Build history of the part. All positions in model axes, mm. Face numbers are marked on the shaded views. A direction names the side the tool comes from. Give positions to 0.01 mm unless a question says otherwise; leave off trailing zeros. Write each loop counter-clockwise with the first axis right and the second up, starting at its lowest first coordinate (ties: lowest second). Pieces come first, ordered by that corner, then holes.
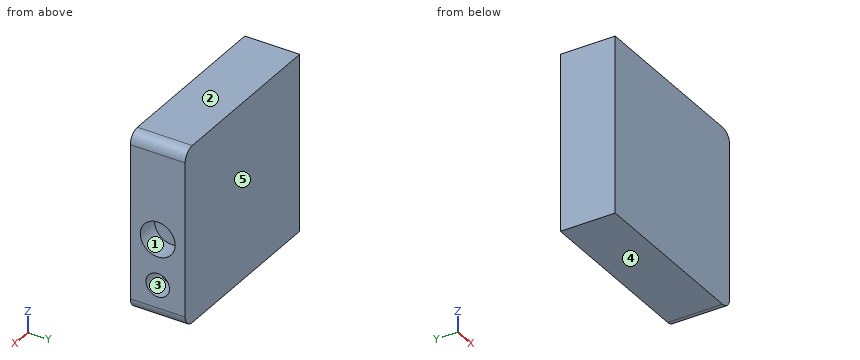
from build123d import *

# Parameters (mm, degrees)
SKETCH1_W           = 80
SKETCH1_H           = 77.5
BOSS_EXTRUDE1_DEPTH = 24
SKETCH2_R           = 5.125
SKETCH2_R_2         = 7.625
CUT_EXTRUDE1_DEPTH  = 10
FILLET1_R           = 5


with BuildPart() as part:
    # Sketch1 → Boss-Extrude1 (new body)
    with BuildSketch(Plane(origin=(0, 0, 0), x_dir=(1, 0, 0), z_dir=(0, 1, 0))):
        with Locations((40, 38.75)):
            Rectangle(SKETCH1_W, SKETCH1_H)
    extrude(amount=BOSS_EXTRUDE1_DEPTH)

    # Sketch2 → Cut-Extrude1 (cut)
    with BuildSketch(Plane(origin=(80, 0, 0), x_dir=(0, 0, -1), z_dir=(1, 0, 0))):
        with Locations((62.5, 12)):
            Circle(SKETCH2_R)
        with Locations((42.5, 12)):
            Circle(SKETCH2_R_2)
    extrude(amount=-CUT_EXTRUDE1_DEPTH, mode=Mode.SUBTRACT)

    # Fillet1
    fillet1_edges = [part.edges().sort_by_distance(p)[0] for p in [
        (80, 12, -77.5),
        (80, 12, 0),
    ]]
    fillet(fillet1_edges, radius=FILLET1_R)


solid = part.part
1. Saw through at B-B on z = -62.5. Give the cut face in (x, y) (3 decimals).
2. Drop a flat-ended pin along its axis: pin 1 (4.5 mm diameter, centred on y = 14, z = -41.5, fed in from +X). Give the stop position or say it passes through.
3. Saw through at C-C on z = -42.5. Give the cut face in (x, y) (3 decimals), plus the area to 3 significant figures.
4. Saw through at A-A on y = 12. Give the cut face in (x, z) (3 decimals).
5. Drill centre lines: line 1 along Y through (x, z) = (75, -42); line 2 along Y through (x, z) = (73, -62.5) (3 decimals); line 3 along X through (y, z) = (15.75, -39). Where is each one in solid material? Low to high.
6. 3-axis set-ups, long thin cutter, end or side, ignore diameter. For the marked faces 1 and 2: which of +Z, -Z, +X, -X, +Y, -Y reach the whole face in a straight line?
7. Mould opens along Y. For the marked faces 3, 4 and 5 say: pulls with the +Y half, pulls with the -Y half, needs draft (parallel to the pull), parting line crosses it, or undercut.
Outcome:
1. outline: (0, 0) - (80, 0) - (80, 6.875) - (70, 6.875) - (70, 17.125) - (80, 17.125) - (80, 24) - (0, 24) - close
2. pin 1: stops at x = 70
3. outline: (0, 0) - (80, 0) - (80, 4.375) - (70, 4.375) - (70, 19.625) - (80, 19.625) - (80, 24) - (0, 24) - close
3. area: 1,770 mm2
4. outline: (0, -77.5) - (75, -77.5) arc R5 ccw to (80, -72.5) - (80, -67.625) - (70, -67.625) - (70, -57.375) - (80, -57.375) - (80, -50.125) - (70, -50.125) - (70, -34.875) - (80, -34.875) - (80, -5) arc R5 ccw to (75, 0) - (0, 0) - close
5. line 1: y = 0 to 4.39, 19.61 to 24
5. line 2: y = 0 to 6.875, 17.125 to 24
5. line 3: x = 0 to 70
6. face 1: +X
6. face 2: +Z, +X, -X, +Y, -Y
7. face 3: undercut
7. face 4: needs draft
7. face 5: pulls with the +Y half
